Autodesk Inventor part; units mm, degrees
ref_plane "YZ Plane" through (0, 0, 0) normal (1, 0, 0) x (0, 1, 0)
ref_plane "XZ Plane" through (0, 0, 0) normal (0, 1, 0) x (-1, 0, 0)
ref_plane "XY Plane" through (0, 0, 0) normal (0, 0, 1) x (1, 0, 0)
sketch "Sketch1" plane through (0, 0, 0) normal (0, 0, 1) x (1, 0, 0)
  line L0 (0, 0) -> (0, 4438.8737)
  line L1 (0, 4438.8737) -> (96, 4438.8737)
  line L2 (96, 4438.8737) -> (196, 0)
  line L3 (196, 0) -> (0, 0)
  circle A0 centre (0, 0) radius 30
  line L4 (0, 1479.6246) -> (162.6667, 1479.6246)
  line L5 (0, 2959.2492) -> (129.3333, 2959.2492)
  circle A1 centre (0, 1479.6246) radius 30
  circle A2 centre (0, 2959.2492) radius 30
  line L6 (186.8761, 405) -> (116.8761, 405)
  line L7 (116.8761, 405) -> (116.8761, 410)
  line L8 (116.8761, 410) -> (186.8761, 410)
  line L9 (186.8761, 410) -> (186.8761, 405)
  line L10 (105.6148, 909.8732) -> (175.6148, 909.8732)
  line L11 (175.6148, 904.8732) -> (105.6148, 904.8732)
  line L12 (105.6148, 904.8732) -> (105.6148, 909.8732)
  line L13 (175.6148, 909.8732) -> (175.6148, 904.8732)
  line L14 (94.3535, 1409.7463) -> (164.3535, 1409.7463)
  line L15 (164.3535, 1404.7463) -> (94.3535, 1404.7463)
  line L16 (94.3535, 1404.7463) -> (94.3535, 1409.7463)
  line L17 (164.3535, 1409.7463) -> (164.3535, 1404.7463)
  line L18 (83.0923, 1909.6195) -> (153.0923, 1909.6195)
  line L19 (153.0923, 1904.6195) -> (83.0923, 1904.6195)
  line L20 (83.0923, 1904.6195) -> (83.0923, 1909.6195)
  line L21 (153.0923, 1909.6195) -> (153.0923, 1904.6195)
  line L22 (71.831, 2409.4927) -> (141.831, 2409.4927)
  line L23 (141.831, 2404.4927) -> (71.831, 2404.4927)
  line L24 (71.831, 2404.4927) -> (71.831, 2409.4927)
  line L25 (141.831, 2409.4927) -> (141.831, 2404.4927)
  line L26 (60.5698, 2909.3658) -> (130.5698, 2909.3658)
  line L27 (130.5698, 2904.3658) -> (60.5698, 2904.3658)
  line L28 (60.5698, 2904.3658) -> (60.5698, 2909.3658)
  line L29 (130.5698, 2909.3658) -> (130.5698, 2904.3658)
  line L30 (49.3085, 3409.239) -> (119.3085, 3409.239)
  line L31 (119.3085, 3404.239) -> (49.3085, 3404.239)
  line L32 (49.3085, 3404.239) -> (49.3085, 3409.239)
  line L33 (119.3085, 3409.239) -> (119.3085, 3404.239)
  line L34 (38.0472, 3909.1122) -> (108.0472, 3909.1122)
  line L35 (108.0472, 3904.1122) -> (38.0472, 3904.1122)
  line L36 (38.0472, 3904.1122) -> (38.0472, 3909.1122)
  line L37 (108.0472, 3909.1122) -> (108.0472, 3904.1122)
  line L38 (0, 1629.6246) -> (159.2874, 1629.6246)
  line L39 (0, 3079.2492) -> (126.6299, 3079.2492)
  point P0 (30, 2959.2492)
  point P1 (0, 2929.2492)
  point P2 (0, 1509.6246)
  point P3 (0, 1449.6246)
  point P4 (0, 30)
  point P5 (30, 0)
  point P6 (186.7634, 410)
  point P7 (175.5022, 909.8732)
  point P8 (164.2409, 1409.7463)
  point P9 (30, 1479.6246)
  point P10 (153.0923, 1904.6195)
  point P11 (152.9796, 1909.6195)
  point P12 (141.831, 2404.4927)
  point P13 (141.7184, 2409.4927)
  point P14 (130.5698, 2904.3658)
  point P15 (130.4571, 2909.3658)
  point P16 (0, 2989.2492)
  point P17 (119.3085, 3404.239)
  point P18 (119.1959, 3409.239)
  point P19 (108.0472, 3904.1122)
  point P20 (107.9346, 3909.1122)
  dimension "d65" = 96
  dimension "d67" = 196
  dimension "d68" = 60
  dimension "d69" = 1480
  dimension "d70" = 1480
  dimension "d71" = 1480
  dimension "d72" = 5
  dimension "d73" = 70
  dimension "d74" = 410
  dimension "d77" = 500
  dimension "d82" = 120
  dimension "d83" = 150
extrude "Plate3" add sketch "Sketch1" along normal blind 4 contours L39 L2 L5 A2 L0 | L0 L1 L2 L34 L36 L35 L30 L32 L31 L39
chamfer "Corner Chamfer2" distance 3 angle 45 4 edges at (119.3085, 3404.239, 2) (119.1959, 3409.239, 2) (108.0472, 3904.1122, 2) (107.9346, 3909.1122, 2)
equation "\"BendRadius\" = Thickness"
equation "\"BendReliefWidth\" = Thickness"
equation "\"BendReliefDepth\" = 0.5 * Thickness"
equation "\"CornerReliefSize\" = 4 * Thickness"
equation "\"MinimumRemnant\" = 2 * Thickness"
equation "\"TransitionRadius\" = BendRadius"
equation "\"JacobiRadiusSize\" = BendRadius"
equation "\"GapSize\" = Thickness"
properties part number "GBK 3301 Center third rib" material "Steel"
The listing builds one solid part. Answer for the finished solid, in the listing's coordinates (mm). Give positions to 0.01 mm unless a question says otherwise; leave off trailing zeros. Order: outer loops, then holes, each group sorted by start corner. A loop starts at its lowest first (then second) coordinate and runs counter-clockwise, first axis right, second up. Notation, with made-up numbers: (14, -37.75) - (57, -37.75) arc R26 ccw to (57, -4.75) - close; hole circle Ø4 at (73, 78). An arc over 180 degrees is marked (long way). One line per item, written item: value. Start each with the question number.
1) A cutting plane is placed at B-B on y = 3868.5. Give the vertices of the cut face in (x, z), then the cut area to 3 significant figures.
2) A cutting plane is placed at A-A on z = 1.5. Give the vertices of the cut face in (x, y).
3) Given pin 1 Ø1.2 at (y, z) = (3907, 2.5) entering from +X, flat-ended and moving along its own axis, determine where the tip first touches the part or whether it passes through.
4) Find the intervals of material crossed by L1, parallel to Y at x = 51.5, z = 3.65; L2, parallel to X at y = 3386, z = 0.3; L3, parallel to X at y = 4271, z = 1.95, in increasing order.
5) A cutting plane is placed at C-C on x = 17.5. Give the vertices of the cut face in (y, z).
Answer sheet:
1. outline: (0, 0) - (108.85, 0) - (108.85, 4) - (0, 4) - close
1. area: 435 mm2
2. outline: (0, 2989.25) arc R30 cw to (30, 2959.25) - (129.33, 2959.25) - (119.38, 3401.24) - (116.31, 3404.24) - (49.31, 3404.24) - (49.31, 3409.24) - (116.2, 3409.24) - (119.13, 3412.24) - (108.11, 3901.11) - (105.05, 3904.11) - (38.05, 3904.11) - (38.05, 3909.11) - (104.93, 3909.11) - (107.87, 3912.11) - (96, 4438.87) - (0, 4438.87) - close
3. pin 1: stops at x = 38.05
4. L1: y = 2959.25 to 3404.24, 3409.24 to 3904.11, 3909.11 to 4438.87
4. L2: x = 0 to 119.72
4. L3: x = 0 to 99.78
5. outline: (2983.62, 0) - (4438.87, 0) - (4438.87, 4) - (2983.62, 4) - close
